```python
from build123d import *

# Parameters (mm, degrees)
SKETCH1_R           = 1
BOSS_EXTRUDE1_DEPTH = 5
SKETCH2_W           = 5
SKETCH2_H           = 40
BOSS_EXTRUDE2_DEPTH = 80
SKETCH3_R           = 2.22
CUT_EXTRUDE3_DEPTH  = 80
BOSS_EXTRUDE5_DEPTH = 5
SKETCH9_W           = 20
SKETCH9_H           = 6
CUT_EXTRUDE7_DEPTH  = 10
SKETCH10_W          = 5
SKETCH10_H          = 8
BOSS_EXTRUDE6_DEPTH = 10
SKETCH11_R          = 1
CUT_EXTRUDE9_DEPTH  = 8
SKETCH12_R          = 1
CUT_EXTRUDE10_DEPTH = 8
SKETCH5_R           = 2.22
BOSS_EXTRUDE7_DEPTH = 5
SKETCH14_R          = 10.2
BOSS_EXTRUDE8_DEPTH = 5


with BuildPart() as part:
    # Sketch1 → Boss-Extrude1 (new body)
    with BuildSketch(Plane(origin=(0, 0, 0), x_dir=(1, 0, 0), z_dir=(0, 1, 0))):
        with BuildLine():
            Line((5.319641756, -11.332905968), (15.319641756, -11.332905968))
            Line((15.319641756, -11.332905968), (15.319641756, 28.667094032))
            Line((15.319641756, 28.667094032), (5.319641756, 28.667094032))
            ThreePointArc((5.319641756, 28.667094032), (-1.751426056, 25.738161844), (-4.680358244, 18.667094032))
            Line((-4.680358244, 18.667094032), (-4.680358244, -1.332905968))
            ThreePointArc((-4.680358244, -1.332905968), (-1.751426056, -8.40397378), (5.319641756, -11.332905968))
        make_face()
        with Locations((5.319641756, 18.667094032)):
            Circle(SKETCH1_R, mode=Mode.SUBTRACT)
        with Locations((5.319641756, -1.332905968)):
            Circle(SKETCH1_R, mode=Mode.SUBTRACT)
    extrude(amount=BOSS_EXTRUDE1_DEPTH)

    # Sketch2 → Boss-Extrude2 (add)
    with BuildSketch(Plane(origin=(0, 5, 0), x_dir=(1, 0, 0), z_dir=(0, 1, 0))):
        with Locations((12.819641756, 8.667094032)):
            Rectangle(SKETCH2_W, SKETCH2_H)
    extrude(amount=BOSS_EXTRUDE2_DEPTH)

    # Sketch3 → Cut-Extrude3 (cut)
    with BuildSketch(Plane.ZY.offset(-10.319641756)):
        with BuildLine():
            ThreePointArc((0.732905968, 35.401978793), (1.440012749, 35.694872012), (1.732905968, 36.401978793))
            Line((1.732905968, 36.401978793), (1.732905968, 69.94419701))
            ThreePointArc((1.732905968, 69.94419701), (1.440012749, 70.651303792), (0.732905968, 70.94419701))
            Line((0.732905968, 70.94419701), (-18.067094032, 70.94419701))
            ThreePointArc((-18.067094032, 70.94419701), (-18.774200813, 70.651303792), (-19.067094032, 69.94419701))
            Line((-19.067094032, 69.94419701), (-19.067094032, 36.401978793))
            ThreePointArc((-19.067094032, 36.401978793), (-18.774200813, 35.694872012), (-18.067094032, 35.401978793))
            Line((-18.067094032, 35.401978793), (0.732905968, 35.401978793))
        make_face()
        with Locations((-13.167094032, 75.54419701)):
            Circle(SKETCH3_R)
        with Locations((-13.167094032, 25.24419701)):
            Circle(SKETCH3_R)
        with Locations((-4.167094032, 25.24419701)):
            Circle(SKETCH3_R)
        with Locations((-4.167094032, 75.54419701)):
            Circle(SKETCH3_R)
    extrude(amount=-CUT_EXTRUDE3_DEPTH, mode=Mode.SUBTRACT)

    # Sketch8 → Boss-Extrude5 (add, through all)
    with BuildSketch(Plane.ZY.offset(-10.319641756)):
        Polygon((-28.667094032, 89.50779106), (-28.667094032, 85), (-16.300533883, 85), (-16.300533883, 94.015582119), align=None)
        Polygon((-1.033654181, 94.015582119), (-1.033654181, 85), (11.332905968, 85), (11.332905968, 89.50779106), align=None)
    extrude(amount=-BOSS_EXTRUDE5_DEPTH)

    # Sketch9 → Cut-Extrude7 (cut)
    with BuildSketch(Plane.ZY.offset(-10.319641756)):
        with Locations((-8.667094032, 13)):
            Rectangle(SKETCH9_W, SKETCH9_H)
    extrude(amount=-CUT_EXTRUDE7_DEPTH, mode=Mode.SUBTRACT)

    # Sketch10 → Boss-Extrude6 (add)
    with BuildSketch(Plane.ZY.offset(-10.319641756)):
        with Locations((-25.767094032, 17.566871705)):
            Rectangle(SKETCH10_W, SKETCH10_H)
        with Locations((8.432905968, 17.566871705)):
            Rectangle(SKETCH10_W, SKETCH10_H)
        with Locations((8.432905968, 75.6)):
            Rectangle(SKETCH10_W, SKETCH10_H)
        with Locations((-25.767094032, 75.6)):
            Rectangle(SKETCH10_W, SKETCH10_H)
    extrude(amount=BOSS_EXTRUDE6_DEPTH)

    # Sketch11 → Cut-Extrude9 (cut)
    with BuildSketch(Plane.XY.offset(10.932905968)):
        with Locations((5.319641756, 17.566871705)):
            Circle(SKETCH11_R)
        with Locations((5.319641756, 75.6)):
            Circle(SKETCH11_R)
    extrude(amount=-CUT_EXTRUDE9_DEPTH, mode=Mode.SUBTRACT)

    # Sketch12 → Cut-Extrude10 (cut)
    with BuildSketch(Plane(origin=(0, 0, -28.267094032), x_dir=(-1, 0, 0), z_dir=(0, 0, -1))):
        with Locations((-5.319641756, 75.6)):
            Circle(SKETCH12_R)
        with Locations((-5.319641756, 17.566871705)):
            Circle(SKETCH12_R)
    extrude(amount=-CUT_EXTRUDE10_DEPTH, mode=Mode.SUBTRACT)

    # Sketch5 → Boss-Extrude7 (add)
    with BuildSketch(Plane(origin=(15.319641756, 0, 0), x_dir=(0, 0, -1), z_dir=(1, 0, 0))):
        with Locations((4.167094032, 25.24419701)):
            Circle(SKETCH5_R)
        with Locations((13.167094032, 25.24419701)):
            Circle(SKETCH5_R)
        with Locations((4.167094032, 75.54419701)):
            Circle(SKETCH5_R)
        with Locations((13.167094032, 75.54419701)):
            Circle(SKETCH5_R)
    extrude(amount=-BOSS_EXTRUDE7_DEPTH)

    # Sketch14 → Boss-Extrude8 (add)
    with BuildSketch(Plane.ZY.offset(-10.319641756)):
        with BuildLine():
            Line((0.732905968, 70.94419701), (-18.067094032, 70.94419701))
            ThreePointArc((-18.067094032, 70.94419701), (-18.774200813, 70.651303792), (-19.067094032, 69.94419701))
            Line((-19.067094032, 69.94419701), (-19.067094032, 36.401978793))
            ThreePointArc((-19.067094032, 36.401978793), (-18.774200813, 35.694872012), (-18.067094032, 35.401978793))
            Line((-18.067094032, 35.401978793), (0.732905968, 35.401978793))
            ThreePointArc((0.732905968, 35.401978793), (1.440012749, 35.694872012), (1.732905968, 36.401978793))
            Line((1.732905968, 36.401978793), (1.732905968, 69.94419701))
            ThreePointArc((1.732905968, 69.94419701), (1.440012749, 70.651303792), (0.732905968, 70.94419701))
        make_face()
        with Locations((-8.667094032, 60.54)):
            Circle(SKETCH14_R, mode=Mode.SUBTRACT)
    extrude(amount=-BOSS_EXTRUDE8_DEPTH)


solid = part.part
```
Input: part model. Units: mm. Frame: model coordinates. A direction names the side the tool comes from. Coordinates: 2 decimals unless noted, no trailing zeros. Loops run counter-clockwise (first coordinate to the right, second up) from the corner with the lowest first, then second, coordinate; pieces in that order, holes last. Notation, with made-up numbers: (-25, -33) - (27, -33) arc R23 ccw to (27, -7) - close; hole circle Ø3 at (56, -14). An arc over 180 degrees is marked (long way). Answer in a Markdown table with one row per item.
(1) Cut plane A-A on y = 60.54. Output: boundary loops of the cut face in (x, z), plus the area to 3 significant figures.
Model answer:
| item | result |
|---|---|
| outline | (10.32, -28.67) - (15.32, -28.67) - (15.32, -18.87) - (10.32, -18.87) - close; (10.32, 1.53) - (15.32, 1.53) - (15.32, 11.33) - (10.32, 11.33) - close |
| area | 98.0 mm² |
(2) Material intervals for L1, parallel to Z at x = 13.75, y = 87; L2, parallel to Y at x = 11.5, z = -11.5; L3, parallel to Y at x = 13.75, z = -18, sorted ascending. Write a range as from..to.
Model answer:
| item | result |
|---|---|
| L1 | z = -28.67..-16.3, -1.03..11.33 |
| L2 | y = 0..10, 16..50.74, 70.34..85 |
| L3 | y = 0..10, 16..56.42, 64.66..93.4 |
(3) Set-up query: faces 1 (the face through (4, 76, 10.933)), 2 (the face through (5, 13.567, 8)), 3 (the face through (13, 89, -16.301)). Return all of +Z, -Z, +X, -X, +Y, -Y with unobstructed straight access to the full face (end or side cutting, diameter ignored); none if empty.
Model answer:
| item | result |
|---|---|
| face 1 | +Z, -X, +Y |
| face 2 | +Z, -Z, -X |
| face 3 | +X, -X, +Y |
(4) Mould query, pull axis Y, two halves, no side actions, for faces 4 (the face through (4.86, 74.71, -25.8)), 5 (the face through (0.32, 18, 8)), 6 (the face through (12.785, 91.793, -22.397)). Classes: pulls with the +Y half, pulls with the -Y half, needs draft (parallel to the pull), parting line crosses it, or undercut.
Model answer:
| item | result |
|---|---|
| face 4 | undercut |
| face 5 | needs draft |
| face 6 | pulls with the +Y half |
(5) Cut plane B-B on x = 12. Output: boundary loops of the cut face in (y, z).
Model answer:
| item | result |
|---|---|
| outline | (0, -28.67) - (89.51, -28.67) - (94.02, -16.3) - (85, -16.3) - (85, -1.03) - (94.02, -1.03) - (89.51, 11.33) - (0, 11.33) - close; hole (10, -18.67) - (16, -18.67) - (16, 1.33) - (10, 1.33) - close; hole circle Ø20.4 at (60.54, -8.67) |
(6) Pin query (flat end, axial travel): P1, Ø6.5, axis at x = 3.5, y = 16.5, coming from the -Z side; P2, Ø4, axis at x = 7.5, y = 18.5, coming from the +Z side; P3, Ø10, axis at y = 79, z = -15, coming from the -X side. Return the tip coordinate at first contact, or that it passes through.
Model answer:
| item | result |
|---|---|
| P1 | stops at z = -28.27 |
| P2 | stops at z = 10.93 |
| P3 | stops at x = 10.32 |
(7) Cut plane C-C on y = 75.6. Output: boundary loops of the cut face in (x, z).
Model answer:
| item | result |
|---|---|
| outline | (0.32, -28.27) - (4.32, -28.27) - (4.32, -23.27) - (0.32, -23.27) - close; (0.32, 5.93) - (4.32, 5.93) - (4.32, 10.93) - (0.32, 10.93) - close; (6.32, -28.27) - (10.32, -28.27) - (10.32, -28.67) - (15.32, -28.67) - (15.32, 11.33) - (10.32, 11.33) - (10.32, 10.93) - (6.32, 10.93) - (6.32, 5.93) - (10.32, 5.93) - (10.32, -23.27) - (6.32, -23.27) - close |
(8) Cut plane D-D on z = -25. Output: boundary loops of the cut face in (x, y).
Model answer:
| item | result |
|---|---|
| outline | (-2.42, 0) - (15.32, 0) - (15.32, 90.84) - (10.32, 90.84) - (10.32, 79.6) - (0.32, 79.6) - (0.32, 71.6) - (10.32, 71.6) - (10.32, 21.57) - (0.32, 21.57) - (0.32, 13.57) - (10.32, 13.57) - (10.32, 5) - (-2.42, 5) - close; hole circle Ø2 at (5.32, 17.57); hole circle Ø2 at (5.32, 75.6) |
